For this review, use the dimensioned drawing (mm, ordinates from the lowest corner) and the shaded views. Give positions to 0.01 mm unless a question says otherwise; leave off trailing zeros. Loops run counter-clockwise (first coordinate to the right, second up) from the corner with the lowest first, then second, coordinate; pieces in that order, holes last. Notation, with made-up numbers: (63, -31.5) - (75, -31.5) arc R21 ccw to (75, 3.5) - close; hole circle Ø11 at (-33, 80.5). An arc over 180 degrees is marked (long way). Put each result on its own line as item: value.
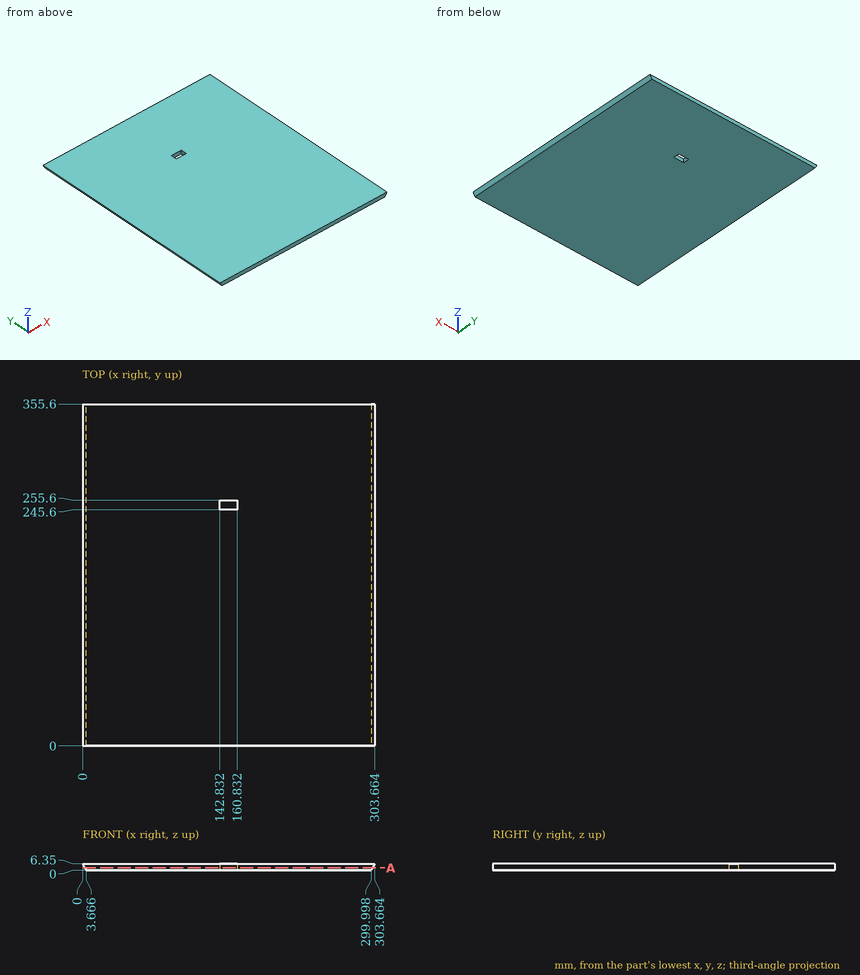
1) Insertion check: pin 1 Ø1.5 at (y, z) = (55, 4) entering from +X. The pin has a flat end and moves straight along its axis. Give the tip position at first contact, or say it passes through.
Geometry check:
pin 1: stops at x = 302.74
2) Wall thickness on line 1 (X direction, y = 304, z = 1) (1 decimal); line 2 (X direction, y = 327.5, z = 2.5); line 3 (X direction, y = 246, z = 3) (1 decimal): over which ranges is each line inside the solid? List them lowest first.
Geometry check:
line 1: x = 3.1 to 300.6
line 2: x = 2.22 to 301.44
line 3: x = 1.9 to 142.8, 160.8 to 301.7
3) Take a section at A-A on z = 2.25. State the section outline as (x, y) points.
Geometry check:
outline: (2.37, 0) - (301.3, 0) - (301.3, 355.6) - (2.37, 355.6) - close; hole (142.83, 245.6) - (160.83, 245.6) - (160.83, 255.6) - (142.83, 255.6) - close
